Input: part model. Units: mm. Frame: model coordinates. Give positions to 0.01 mm unless a question says otherwise; leave off trailing zeros. Loops run counter-clockwise (first coordinate to the right, second up) from the corner with the lowest first, then second, coordinate; pieces in that order, holes last.
from build123d import *

# Parameters (mm, degrees)
SKETCH1_W           = 50
SKETCH1_H           = 70
BOSS_EXTRUDE1_DEPTH = 5
SKETCH2_R           = 1.6
CUT_EXTRUDE1_DEPTH  = 10


with BuildPart() as part:
    # Sketch1 → Boss-Extrude1 (new body)
    with BuildSketch(Plane(origin=(0, 0, 0), x_dir=(1, 0, 0), z_dir=(0, 1, 0))):
        with Locations((-9.575074469, 8.274395374)):
            Rectangle(SKETCH1_W, SKETCH1_H)
        with BuildLine():
            Line((-26.595889749, 32.545210655), (7.445740812, 32.545210655))
            ThreePointArc((7.445740812, 32.545210655), (9.695740812, 30.295210655), (7.445740812, 28.045210655))
            Line((7.445740812, 28.045210655), (-26.595889749, 28.045210655))
            ThreePointArc((-26.595889749, 28.045210655), (-28.845889749, 30.295210655), (-26.595889749, 32.545210655))
        make_face(mode=Mode.SUBTRACT)
        with BuildLine():
            Line((-14.575074469, 23.274395374), (-4.575074469, 23.274395374))
            ThreePointArc((-4.575074469, 23.274395374), (0.424925531, 18.274395374), (-4.575074469, 13.274395374))
            Line((-4.575074469, 13.274395374), (-14.575074469, 13.274395374))
            ThreePointArc((-14.575074469, 13.274395374), (-19.575074469, 18.274395374), (-14.575074469, 23.274395374))
        make_face(mode=Mode.SUBTRACT)
        with BuildLine():
            Line((-26.595889749, 4.003580094), (7.445740812, 4.003580094))
            ThreePointArc((7.445740812, 4.003580094), (9.695740812, 6.253580094), (7.445740812, 8.503580094))
            Line((7.445740812, 8.503580094), (-26.595889749, 8.503580094))
            ThreePointArc((-26.595889749, 8.503580094), (-28.845889749, 6.253580094), (-26.595889749, 4.003580094))
        make_face(mode=Mode.SUBTRACT)
    extrude(amount=BOSS_EXTRUDE1_DEPTH)

    # Sketch2 → Cut-Extrude1 (cut)
    with BuildSketch(Plane.XY.offset(26.725604626)):
        with Locations((-9.575074469, 2.5)):
            Circle(SKETCH2_R)
        with Locations((-24.575074469, 2.5)):
            Circle(SKETCH2_R)
        with Locations((5.424925531, 2.5)):
            Circle(SKETCH2_R)
    extrude(amount=-CUT_EXTRUDE1_DEPTH, mode=Mode.SUBTRACT)


solid = part.part
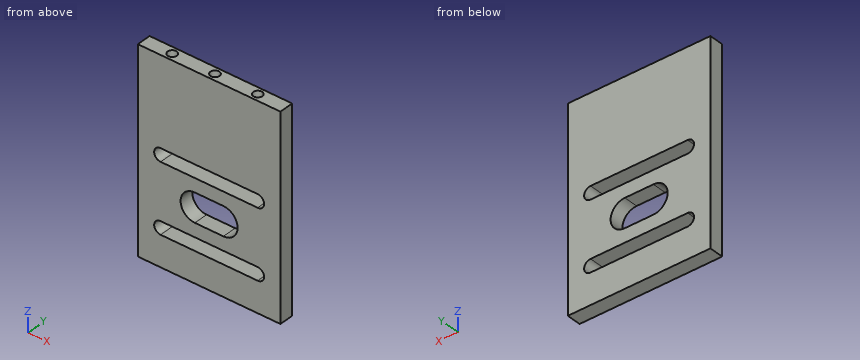
(1) Cut plane A-A (x = -12.5). Return the cut outline in (y, z).
Values follow:
outline: (0, -43.27) - (5, -43.27) - (5, -32.55) - (0, -32.55) - close; (0, -28.05) - (5, -28.05) - (5, -23.27) - (0, -23.27) - close; (0, -13.27) - (5, -13.27) - (5, -8.5) - (0, -8.5) - close; (0, -4) - (5, -4) - (5, 26.73) - (0, 26.73) - close
(2) Pin query (flat end, axial travel): pin 1 Ø1 at (x, y) = (5, 2.5) entering from +Z. Return the tip coordinate at first contact, or that it passes through.
Values follow:
pin 1: stops at z = 16.73
(3) Cut plane C-C (y = 2.5). Return the cut outline in (x, z), and give its area (3 significant figures).
Values follow:
outline: (-34.58, -43.27) - (15.42, -43.27) - (15.42, 26.73) - (7.02, 26.73) - (7.02, 16.73) - (3.82, 16.73) - (3.82, 26.73) - (-7.98, 26.73) - (-7.98, 16.73) - (-11.18, 16.73) - (-11.18, 26.73) - (-22.98, 26.73) - (-22.98, 16.73) - (-26.18, 16.73) - (-26.18, 26.73) - (-34.58, 26.73) - close; hole (-26.6, -32.55) - (7.45, -32.55) arc R2.25 ccw to (7.45, -28.05) - (-26.6, -28.05) arc R2.25 ccw to start; hole (-26.6, -8.5) - (7.45, -8.5) arc R2.25 ccw to (7.45, -4) - (-26.6, -4) arc R2.25 ccw to start; hole (-14.58, -23.27) - (-4.58, -23.27) arc R5 ccw to (-4.58, -13.27) - (-14.58, -13.27) arc R5 ccw to start
area: 2,890 mm2
(4) Ray query, probe 1 along Z at (x, y) = (-26, 2.7); probe 2 along Z at (x, y) = (-12, 1.25); probe 3 along Z at (x, y) = (-23, 4.5). Return the intervals inside material, ascending.
Values follow:
probe 1: z = -43.27 to -32.55, -28.05 to -8.5, -4 to 16.73
probe 2: z = -43.27 to -32.55, -28.05 to -23.27, -13.27 to -8.5, -4 to 26.73
probe 3: z = -43.27 to -32.55, -28.05 to -8.5, -4 to 26.73
(5) Cut plane B-B (x = 2). Return the cut outline in (y, z), and give its area (3 significant figures).
Values follow:
outline: (0, -43.27) - (5, -43.27) - (5, -32.55) - (0, -32.55) - close; (0, -28.05) - (5, -28.05) - (5, -8.5) - (0, -8.5) - close; (0, -4) - (5, -4) - (5, 26.73) - (0, 26.73) - close
area: 305 mm2
(6) Cut plane D-D (z = -21.5). Return the cut outline in (x, y), and give its area (3 significant figures).
Values follow:
outline: (-34.58, 0) - (-18.4, 0) - (-18.4, 5) - (-34.58, 5) - close; (-0.75, 0) - (15.42, 0) - (15.42, 5) - (-0.75, 5) - close
area: 162 mm2
